Autodesk Inventor part; units mm, degrees
ref_plane "Work Plane1" through (0, 5.25, 0) normal (0, 1, 0) x (-1, 0, 0)
ref_plane "YZ Plane" through (0, 0, 0) normal (1, 0, 0) x (0, 1, 0)
ref_plane "XY Plane" through (0, 0, 0) normal (0, 0, 1) x (1, 0, 0)
sketch "Sketch1" plane through (0, 0, 0) normal (0, 0, 1) x (1, 0, 0)
  circle A0 centre (0, 0) radius 16
  line L0 (0, 0) -> (0, 8.955)
  circle A1 centre (0, 0) radius 8.955
  dimension "d0" = 32
  dimension "d1" = 8.955
extrude "Extrusion1" add sketch "Sketch1" against normal blind 1 contours A0 | A1
extrude "Extrusion2" add sketch "Sketch1" against normal blind 7 contours A1
sketch "Sketch2" plane through (0, 0, -7) normal (0, 0, -1) x (-1, 0, 0)
  circle A0 centre (0, 0) radius 8.455
  dimension "d6" = 16.91
extrude "Extrusion3" cut sketch "Sketch2" against normal blind 5
sketch "Sketch3" plane through (0, 0, 0) normal (0, 0, 1) x (1, 0, 0)
  circle A0 centre (0, 0) radius 5
  dimension "d9" = 10
extrude "Extrusion4" add sketch "Sketch3" along normal blind 15
sketch "Sketch4" plane through (0, 0, 15) normal (0, 0, 1) x (1, 0, 0)
  line L0 (-2, 2) -> (2, 2)
  line L1 (2, 2) -> (2, -2)
  line L2 (2, -2) -> (-2, -2)
  line L3 (-2, -2) -> (-2, 2)
  line L4 (-2, 2) -> (2, -2) construction
  line L5 (2, 2) -> (-2, -2) construction
  point P0 (0, 0)
  dimension "d12" = 4
  dimension "d13" = 4
extrude "Extrusion5" cut sketch "Sketch4" against normal through all
ref_plane "Work Plane1" through (0, 5.25, 0) normal (0, 1, 0) x (-1, 0, 0)
sketch "Sketch5" plane through (0, 5.25, 0) normal (0, 1, 0) x (-1, 0, 0)
  circle A0 centre (0, 7.5) radius 1.5
  point P0 (0, 0)
  dimension "d17" = 3
extrude "Extrusion6" cut sketch "Sketch5" against normal through all
thread "Thread1"
thread "Thread2"
sketch "Sketch7" plane through (0, 0, -1) normal (0, 0, -1) x (-1, 0, 0)
  circle A0 centre (0, 0) radius 5
  line L0 (0, 0) -> (8.4853, 8.4853)
  line L1 (0, 0) -> (12, 0) construction
  circle A1 centre (8.4853, 8.4853) radius 1.5
  dimension "d24" = 12
  dimension "d25" = 45
  dimension "d26" = 3
extrude "Extrusion7" cut sketch "Sketch7" against normal through all contours A1
thread "Thread3"
pattern_circular "Circular Pattern1" count 4 over 360 about axis through (0, 0, 0) along (0, 0, -1) of "Extrusion7"
thread "Thread4"
thread "Thread5"
thread "Thread6"
properties part number "tuk-tukan" material "Stainless Steel"
Model file for the job. Use its own axes, mm. A direction names the side the tool comes from. Give positions to 0.01 mm unless a question says otherwise; leave off trailing zeros. Order: outer loops, then holes, each group sorted by start corner. A loop starts at its lowest first (then second) coordinate and runs counter-clockwise, first axis right, second up.
1) Wall check: probe 1 along Z at (x, y) = (0, 4); probe 2 along Z at (x, y) = (2.5, 12); probe 3 along X at (y, z) = (1, 9.5). Give the ranges that are in metal, low to high.
2) Saw through at B-B, the plane x = 0. Write the cut outline in (y, z) (3 decimals), then the cut area to 3 significant figures.
3) Saw through at A-A, the plane y = 0. Write the cut outline in (x, z) (3 decimals), then the cut area to 3 significant figures.
4) Saw through at C-C, the plane z = 11.5. Write the cut outline in (x, y), then the cut area to 3 significant figures.
5) Saw through at D-D, the plane x = -9.5. Write the cut outline in (y, z), then the cut area to 3 significant figures.
6) Mould opens along Y. For faces 1 (the cylindrical face through (1.5, 3.52, 7.57)), 2 (the cylindrical face through (4.77, -1.5, 7.4)), 3 (the cylindrical face through (8.16, -7.02, -0.51)), 4 (the cylindrical face through (-7.02, -8.16, -0.51)) say: +Y half, -Y half, draft (parallel to the pull), parting line (faces both ways), or undercut.
7) 3-axis set-ups, long thin cutter, end or side, ignore diameter. For faces 5 (the flat face through (-1.4, 2, 6.6)), 6 (the flat face through (-4, 4, 0)), 7 (the flat face through (7, -7, -1)): which of +Z, -Z, +X, -X, +Y, -Y reach the whole face in a straight line?
8) Pin check, flat tips, straight feed: pin 1 (2 mm diameter, centred on y = -11, z = -4.5, fed in from -X); pin 2 (5 mm diameter, centred on x = 3, z = 8, fed in from -Y); pin 3 (1 mm diameter, centred on x = 6.5, y = -4.5, fed in from -Z); pin 4 (1.2 mm diameter, centred on y = 0.5, z = 4, fed in from +X). Stop position of each tip, or through.
Computed:
1. probe 1: z = -2 to 6, 9 to 15
1. probe 2: z = -1 to 0
1. probe 3: x = -4.9 to -2, 2 to 4.9
2. outline: (-16, -1) - (-8.955, -1) - (-8.955, -7) - (-8.455, -7) - (-8.455, -2) - (-2, -2) - (-2, 6) - (-5, 6) - (-5, 0) - (-16, 0) - close; (-5, 9) - (-2, 9) - (-2, 15) - (-5, 15) - close; (2, -2) - (8.455, -2) - (8.455, -7) - (8.955, -7) - (8.955, -1) - (16, -1) - (16, 0) - (5, 0) - (5, 6) - (2, 6) - close; (2, 9) - (5, 9) - (5, 15) - (2, 15) - close
2. area: 119 mm2
3. outline: (-16, -1) - (-8.955, -1) - (-8.955, -7) - (-8.455, -7) - (-8.455, -2) - (-2, -2) - (-2, 15) - (-5, 15) - (-5, 0) - (-16, 0) - close; (2, -2) - (8.455, -2) - (8.455, -7) - (8.955, -7) - (8.955, -1) - (16, -1) - (16, 0) - (5, 0) - (5, 15) - (2, 15) - close
3. area: 137 mm2
4. outline: circle Ø10 at (0, 0); hole (-2, -2) - (2, -2) - (2, 2) - (-2, 2) - close
4. area: 62.5 mm2
5. outline: (-12.87, -1) - (-9.59, -1) - (-9.59, 0) - (-12.87, 0) - close; (-7.38, -1) - (7.38, -1) - (7.38, 0) - (-7.38, 0) - close; (9.59, -1) - (12.87, -1) - (12.87, 0) - (9.59, 0) - close
5. area: 21.3 mm2
6. face 1: draft
6. face 2: parting line
6. face 3: undercut
6. face 4: undercut
7. face 5: +Z, -Z
7. face 6: +Z
7. face 7: -Z
8. pin 1: passes through
8. pin 2: stops at y = -4.96
8. pin 3: stops at z = -2
8. pin 4: stops at x = 5
